Work out the finished part from the listing and answer in its coordinate system (mm). A direction names the side the tool comes from. Give positions to 0.01 mm unless a question says otherwise; leave off trailing zeros. Loops run counter-clockwise (first coordinate to the right, second up) from the corner with the lowest first, then second, coordinate; pieces in that order, holes last. Notation, with made-up numbers: M 84,62.25 L 91,62.25 A5 ccw 91,67.25 Z; hole C 75.25,46.5 d6. An arc over 180 degrees is marked long. Answer as a JSON object with one key per item and string values. Group by question number.
```python
from build123d import *

# Parameters (mm, degrees)
BASPROSKE_W             = 7.5
BASPROSKE_H             = 4.5
TOOTHCUT_DEPTH          = 10.836157786
TEETHCUTS_COUNT         = 16
TEETHCUTS_ANGLE         = 337.5
BORSKE_R                = 2.5
BORE_DEPTH              = 50.0000508
ESQUISSE4_R             = 6
BOSS_EXTRU_3_DEPTH      = 1
ESQUISSE5_R             = 6.027848577
ESQUISSE5_R_2           = 2.85
BOSS_EXTRU_4_DEPTH      = 1
ESQUISSE7_R             = 3.00711341
BOSS_EXTRU_6_DEPTH      = 8.5
ESQUISSE9_R             = 13.75
ESQUISSE9_R_2           = 5.5
BOSS_EXTRU_8_DEPTH      = 2
ESQUISSE10_R            = 1.5
ENL_V_MAT_EXTRU_3_DEPTH = 23.591480695
ESQUISSE11_R            = 3
ENL_V_MAT_EXTRU_4_DEPTH = 4
BOSS_EXTRU_9_START      = 4
ESQUISSE12_R            = 3
BOSS_EXTRU_9_DEPTH      = 4
ESQUISSE13_R            = 5.5
BOSS_EXTRU_10_DEPTH     = 2
ESQUISSE16_R            = 8
BOSS_EXTRU_11_DEPTH     = 1
ESQUISSE14_R            = 6
ENL_V_MAT_EXTRU_5_DEPTH = 1.5
ESQUISSE15_R            = 3.25
ENL_V_MAT_EXTRU_6_DEPTH = 4.5


with BuildPart() as part:
    # BasProSke → Base-Revolve (revolve)
    with BuildSketch(Plane(origin=(0, 0, 0), x_dir=(1, 0, 0), z_dir=(0, 1, 0)), mode=Mode.PRIVATE) as base_revolve_sk:
        with Locations((3.75, 2.25)):
            Rectangle(BASPROSKE_W, BASPROSKE_H)
    revolve(base_revolve_sk.sketch.rotate(Axis((-10, 0, 0), (1, 0, 0)), 180), axis=Axis((-10, 0, 0), (1, 0, 0)))

    # TooCutSke → ToothCut (cut, through all)
    with BuildSketch(Plane(origin=(0, 0, 0), x_dir=(0, 0, -1), z_dir=(1, 0, 0))):
        with BuildLine():
            ThreePointArc((0.306025637, 3.360092902), (0, 3.374), (-0.306025637, 3.360092902))
            ThreePointArc((-0.306025637, 3.360092902), (-0.415941512, 3.953968919), (-0.738171669, 4.464789776))
            ThreePointArc((-0.738171669, 4.464789776), (0, 4.5254), (0.738171669, 4.464789776))
            ThreePointArc((0.738171669, 4.464789776), (0.415941512, 3.953968919), (0.306025637, 3.360092902))
        make_face()
    toothcut = extrude(amount=TOOTHCUT_DEPTH, mode=Mode.SUBTRACT)

    # TeethCuts: ToothCut ×16 about axis
    teethcuts_axis = Axis((-10, 0, 0), (1, 0, 0))
    for i in range(1, TEETHCUTS_COUNT):
        add(toothcut.rotate(teethcuts_axis, i * TEETHCUTS_ANGLE / (TEETHCUTS_COUNT - 1)), mode=Mode.SUBTRACT)

    # BorSke → Bore (cut, symmetric)
    with BuildSketch(Plane(origin=(0, 0, 0), x_dir=(0, 0, -1), z_dir=(1, 0, 0))):
        with Locations(Location((0, 0, 0), (0, 0, 180))):
            Circle(BORSKE_R)
    extrude(amount=BORE_DEPTH, both=True, mode=Mode.SUBTRACT)

    # Esquisse4 → Boss.-Extru.3 (add)
    with BuildSketch(Plane.ZY):
        Circle(ESQUISSE4_R)
    extrude(amount=BOSS_EXTRU_3_DEPTH)

    # Esquisse5 → Boss.-Extru.4 (add)
    with BuildSketch(Plane(origin=(7.5, 0, 0), x_dir=(0, 0, -1), z_dir=(1, 0, 0))):
        Circle(ESQUISSE5_R)
        Circle(ESQUISSE5_R_2, mode=Mode.SUBTRACT)
    extrude(amount=BOSS_EXTRU_4_DEPTH)

    # Esquisse7 → Boss.-Extru.6 (add)
    with BuildSketch(Plane(origin=(0, 0, 0), x_dir=(0, 0, -1), z_dir=(1, 0, 0))):
        Circle(ESQUISSE7_R)
    extrude(amount=BOSS_EXTRU_6_DEPTH)

    # Esquisse9 → Boss.-Extru.8 (add)
    with BuildSketch(Plane.ZY.offset(1)):
        Circle(ESQUISSE9_R)
        Circle(ESQUISSE9_R_2, mode=Mode.SUBTRACT)
    extrude(amount=BOSS_EXTRU_8_DEPTH)

    # Esquisse10 → Enlèv. mat.-Extru.3 (cut, through all)
    with BuildSketch(Plane.ZY.offset(3)):
        with Locations((0, 11.3)):
            Circle(ESQUISSE10_R)
        with Locations((0, -11.3)):
            Circle(ESQUISSE10_R)
    extrude(amount=-ENL_V_MAT_EXTRU_3_DEPTH, mode=Mode.SUBTRACT)

    # Esquisse11 → Enlèv. mat.-Extru.4 (cut)
    with BuildSketch(Plane.ZY.offset(1)):
        Circle(ESQUISSE11_R)
    extrude(amount=-ENL_V_MAT_EXTRU_4_DEPTH, mode=Mode.SUBTRACT)

    # Esquisse12 → Boss.-Extru.9 (add)
    with BuildSketch(Plane.ZY.offset(-3).offset(BOSS_EXTRU_9_START)):
        Circle(ESQUISSE12_R)
    extrude(amount=-BOSS_EXTRU_9_DEPTH)

    # Esquisse13 → Boss.-Extru.10 (add)
    with BuildSketch(Plane.ZY.offset(1)):
        Circle(ESQUISSE13_R)
    extrude(amount=BOSS_EXTRU_10_DEPTH)

    # Esquisse16 → Boss.-Extru.11 (add)
    with BuildSketch(Plane(origin=(-1, 0, 0), x_dir=(0, 0, -1), z_dir=(1, 0, 0))):
        with Locations(Location((0, 0, 0), (0, 0, 180))):
            Circle(ESQUISSE16_R)
    extrude(amount=BOSS_EXTRU_11_DEPTH)

    # Esquisse14 → Enlèv. mat.-Extru.5 (cut)
    with BuildSketch(Plane.ZY.offset(3)):
        Circle(ESQUISSE14_R)
    extrude(amount=-ENL_V_MAT_EXTRU_5_DEPTH, mode=Mode.SUBTRACT)

    # Esquisse15 → Enlèv. mat.-Extru.6 (cut)
    with BuildSketch(Plane.ZY.offset(1.5)):
        Circle(ESQUISSE15_R)
    extrude(amount=-ENL_V_MAT_EXTRU_6_DEPTH, mode=Mode.SUBTRACT)


solid = part.part
```
Item 1: A cutting plane is placed at A-A (y = 11.3). Determine the outline of the cut face in (x, z), and give its area (3 significant figures).
Item 2: For a pull along X with two mould halves and no side action, classify faces 5 (the cylindrical face through (7.99, -3.67, 4.78)), 6 (the flat face through (-1, -6, 6)), 7 (the cylindrical face through (3.698, 3.477, 1.881)), 8 (the cylindrical face through (3.698, -0.408, 3.932)) as pulls with the +X half, pulls with the -X half, needs draft (parallel to the pull), parting line crosses it, or undercut.
Item 3: A tool of negligible diameter and unlimited length cuts with its end or side. For faces 1 (the cylindrical face through (-2.014, -12.764, -0.325)), 2 (the flat face through (-1.5, -3, 3)), 3 (the cylindrical face through (3.7, -3.79, 1.13)), 4 (the cylindrical face through (-0.51, 7.81, -1.73)), from which of +Z, -Z, +X, -X, +Y, -Y can it reach the whole face along a straight path? Write none if from no direction.
Item 4: A cutting plane is placed at D-D (z = 9.75). Determine the outline of the cut face in (x, y).
Item 5: Find the intervals of material crossed by probe 1 along X at (y, z) = (4.5, -0.5); probe 2 along X at (y, z) = (-3.25, 8.5); probe 3 along X at (y, z) = (6.5, 1.75), in increasing order. Write a range as [from, to].
Item 6: A cutting plane is placed at B-B (y = 6.5). Determine the outline of the cut face in (x, z), and give its area (3 significant figures).
Item 7: A cutting plane is placed at C-C (z = -10). Determine the outline of the cut face in (x, y), and give its area (3 significant figures).
Item 8: Given pin 1 Ø1.5 at (x, y) = (4.5, 2) entering from -Z; pin 2 Ø1.5 at (y, z) = (9.5, -6) entering from +X; pin 3 Ø2 at (y, z) = (1, 0) entering from -X, each flat-ended and moving along its own axis, determine where each tip first touches the part or whether it passes through.
The answers:
{
 "1": {"outline": "M -3,-7.83 L -1,-7.83 L -1,-1.5 L -3,-1.5 Z; M -3,1.5 L -1,1.5 L -1,7.83 L -3,7.83 Z", "area": "25.3 mm^2"},
 "2": {"face 5": "needs draft", "face 6": "pulls with the +X half", "face 7": "undercut", "face 8": "undercut"},
 "3": {"face 1": "+X, -X", "face 2": "-X", "face 3": "none", "face 4": "+X"},
 "4": {"outline": "M -3,-9.7 L -1,-9.7 L -1,9.7 L -3,9.7 Z"},
 "5": {"probe 1": "x = [-1.5, 0], [7.5, 8.5]", "probe 2": "x = [-3, -1]", "probe 3": "x = [-3, 0]"},
 "6": {"outline": "M -3,-12.12 L -1,-12.12 L -1,-4.66 L 0,-4.66 L 0,4.66 L -1,4.66 L -1,12.12 L -3,12.12 Z", "area": "57.8 mm^2"},
 "7": {"outline": "M -3,-9.44 L -1,-9.44 L -1,9.44 L -3,9.44 Z", "area": "37.7 mm^2"},
 "8": {"pin 1": "stops at z = -3.83", "pin 2": "stops at x = -1", "pin 3": "stops at x = 3"}
}
